Read the model definition and answer for the solid it produces. Units are mm, in the model's axes. Give positions to 0.01 mm unless a question says otherwise; leave off trailing zeros. Order: outer loops, then holes, each group sorted by start corner. A loop starts at its lowest first (then second) coordinate and runs counter-clockwise, first axis right, second up. Notation, with made-up numbers: M -13,-37 L 8,-37 A8 cw 8,-25 Z; hole C 9.25,58 d4. An arc over 180 degrees is marked long. Write item = value, one per line. Start each with the question number.
from build123d import *

# Parameters (mm, degrees)
RESSALTO_EXTRUS_O1_DEPTH = 15
RESSALTO_EXTRUS_O2_DEPTH = 3


with BuildPart() as part:
    # Esboço1 → Ressalto-extrusão1 (new body)
    with BuildSketch(Plane(origin=(0, 0, 0), x_dir=(1, 0, 0), z_dir=(0, 1, 0))):
        Polygon((10.484125197, 87.541408798), (10.657910977, 88.861442851), (-10.689651623, 88.857262857), (-10.515874803, 87.537296858), align=None)
    extrude(amount=RESSALTO_EXTRUS_O1_DEPTH)

    # Esboço2 → Ressalto-extrusão2 (add)
    with BuildSketch(Plane(origin=(-0.017140787, 0, -87.53935258), x_dir=(0.999999981, 0, -0.000195807), z_dir=(0.000195807, 0, 0.999999981))):
        with BuildLine():
            Line((-6.498734217, 6), (-6.498734217, 4))
            ThreePointArc((-6.498734217, 4), (0.001265984, 5.08571975), (6.501266185, 4))
            Line((6.501266185, 4), (6.501266185, 6))
            ThreePointArc((6.501266185, 6), (0.001265984, 8.400658095), (-6.498734217, 6))
        make_face()
    extrude(amount=RESSALTO_EXTRUS_O2_DEPTH)


solid = part.part
1) Find section A-A on y = 4.5. Determine the outline of the cut face in (x, z).
2) Find section B-B on x = 8. Determine the outline of the cut face in (y, z).
3) Find section D-D on y = 11.75. Determine the outline of the cut face in (x, z).
4) Each of these flat-tipped pins is pushed along its axis until it touches: P1, Ø2, axis at y = 8, z = -85.5, coming from the +X side; P2, Ø3, axis at x = -1.5, y = 2.5, coming from the +Z side; P3, Ø0.6, axis at y = 5.5, z = -86.5, coming from the +X side. Where does it stop, or does it pass through?
5) Find the intervals of material crossed by probe 1 along Z at (x, y) = (3.5, 9.5); probe 2 along Z at (x, y) = (-0.75, 7.75); probe 3 along Y at (x, z) = (0.25, -84.95), in increasing order. Write a range as [from, to].
6) Find section C-C on y = 7.75. Determine the outline of the cut face in (x, z).
Numbers:
q1.outline = M -10.69,-88.86 L 10.66,-88.86 L 10.48,-87.54 L 6.48,-87.54 L 6.48,-84.54 L 4.79,-84.54 L 4.79,-87.54 L -4.82,-87.54 L -4.82,-84.54 L -6.52,-84.54 L -6.52,-87.54 L -10.52,-87.54 Z
q2.outline = M 0,-88.86 L 15,-88.86 L 15,-87.54 L 0,-87.54 Z
q3.outline = M -10.69,-88.86 L 10.66,-88.86 L 10.48,-87.54 L -10.52,-87.54 Z
q4.P1 = 5.09
q4.P2 = -87.54
q4.P3 = 6.48
q5.probe_1 = [-88.86, -87.54]
q5.probe_2 = [-88.86, -84.54]
q5.probe_3 = [5.08, 8.4]
q6.outline = M -10.69,-88.86 L 10.66,-88.86 L 10.48,-87.54 L 3.53,-87.54 L 3.53,-84.54 L -3.56,-84.54 L -3.56,-87.54 L -10.52,-87.54 Z
